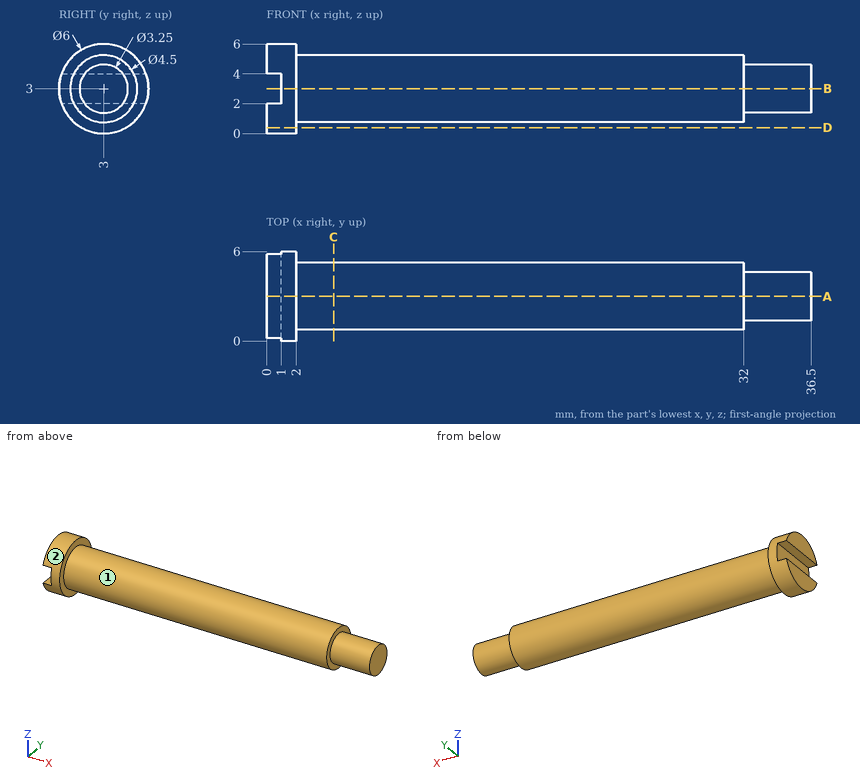
Source: three-view drawing plus pictorial views. Frame: mm from the lowest corner of the part. A direction names the side the tool comes from. Give positions to 0.01 mm unless a question says otherwise; leave off trailing zeros. Order: outer loops, then holes, each group sorted by start corner. A loop starts at its lowest first (then second) coordinate and runs counter-clockwise, first axis right, second up. Notation, with made-up numbers: M 74,-35 L 127,-35 A22 ccw 127,-20 Z; hole C -26.75,-27.75 d9. An arc over 180 degrees is marked long. Return JSON: item names as keys, results as strings.
Item 1: Access query for the marked faces 1 and 2. Directions: +Z, -Z, +X, -X, +Y, -Y. A direction counts if a zero-diameter tool reaches every point of the face in a straight line with its end or side. Return the directions, or none.
Solutions:
{"face 1": "+X", "face 2": "+X, -X"}
Item 2: Cut plane C-C (x = 4.5). Return loops of the section in (y, z), then the cut area to 3 significant figures.
Solutions:
{"outline": "C 3,3 d4.5", "area": "15.9 mm^2"}
Item 3: First-contact query: P1, Ø2, axis at x = 26.5, y = 2.5, coming from the +Z side; P2, Ø3, axis at x = 32, y = 5, coming from the -Z side. Flat tips, straight axial feed; report the tip coordinate or a pass-through.
Solutions:
{"P1": "z = 5.25", "P2": "z = 0.81"}
Item 4: Ray query, probe 1 along X at (y, z) = (0.9, 1.15); probe 2 along X at (y, z) = (2.5, 2.4); probe 3 along Y at (x, z) = (8.5, 2.15). Return the intervals inside material, ascending.
Solutions:
{"probe 1": "0 to 2", "probe 2": "1 to 36.5", "probe 3": "0.92 to 5.08"}
Item 5: Cut plane B-B (z = 3). Return loops of the section in (x, y) (3 decimals).
Solutions:
{"outline": "M 1,0 L 2,0 L 2,0.75 L 32,0.75 L 32,1.375 L 36.5,1.375 L 36.5,4.625 L 32,4.625 L 32,5.25 L 2,5.25 L 2,6 L 1,6 Z"}
Item 6: Cut plane D-D (z = 0.4). Return loops of the section in (x, y), then the cut area to 3 significant figures.
Solutions:
{"outline": "M 0,1.5 L 2,1.5 L 2,4.5 L 0,4.5 Z", "area": "5.99 mm^2"}
Item 7: Cut plane A-A (y = 3). Return loops of the section in (x, z) (3 decimals), then the cut area to 3 significant figures.
Solutions:
{"outline": "M 0,0 L 2,0 L 2,0.75 L 32,0.75 L 32,1.375 L 36.5,1.375 L 36.5,4.625 L 32,4.625 L 32,5.25 L 2,5.25 L 2,6 L 0,6 L 0,4 L 1,4 L 1,2 L 0,2 Z", "area": "160 mm^2"}
